Model file for the job. Use its own axes, mm. Face numbers are marked on the shaded views. Round coordinates to 2 decimals unless told otherwise and drop trailing zeros. Order: outer loops, then holes, each group sorted by start corner. A loop starts at its lowest first (then second) coordinate and runs counter-clockwise, first axis right, second up. Notation, with made-up numbers: (-10.75, 84) -> (21.25, 84) arc R21 ccw to (21.25, 112) -> close; hole circle Ø11 at (64.25, 3). An arc over 180 degrees is marked (long way). Put each result on its own line as item: value. Start each with the question number.
Q1. Pull direction Y, two halves, no side cores. Call the marked faces 1, 2, 3 and 4: released by +Y, released by -Y, zero draft, split by the parting line, or undercut.
Q2. Cut at D-D, the plane z = 47.5. List the corners of the cut face in (x, y), and give its area (3 significant figures).
Q3. Cut at B-B, the plane x = 7.5. List the corners of the cut face in (y, z), and give its area (3 significant figures).
Q4. Cut at A-A, the plane z = 43.25. List the corners of the cut face in (x, y), and give its area (3 significant figures).
Q5. Cut at C-C, the plane y = 3.45. List the corners of the cut face in (x, z).
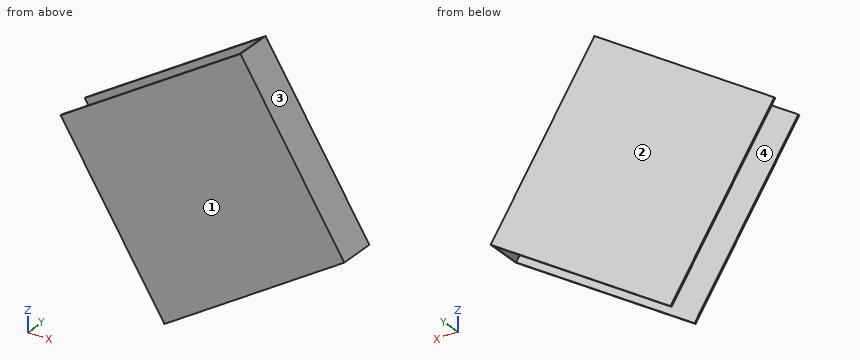
from build123d import *

# Parameters (mm, degrees)
BOX163_W               = 6
BOX163_H               = 6.45
BOX163_DEPTH           = 1.05
BOX162_W               = 6
BOX162_H               = 6.5
BOX162_DEPTH           = 1.15
CUT079_ROLL_ANGLE      = 90
CUT079_PITCH_ANGLE     = -58
CUT079_PLACEMENT_ANGLE = 180


with BuildPart() as small_cu_gnd_electrode068:
    # Box163 → Box163 (new body)
    with BuildSketch(Plane.XY.offset(0.05)):
        with Locations((3, 3.225)):
            Rectangle(BOX163_W, BOX163_H)
    extrude(amount=BOX163_DEPTH)


with BuildPart() as small_cu_electrode002_short_axis_gnd007:
    # Box162 → Box162 (new body)
    with BuildSketch(Plane.XY):
        with Locations((3, 3.25)):
            Rectangle(BOX162_W, BOX162_H)
    extrude(amount=BOX162_DEPTH)

    # Cut079: cut Small Cu GND Electrode068
    add(small_cu_gnd_electrode068.part, mode=Mode.SUBTRACT)


with BuildPart() as small_cu_electrode002_short_axis_gnd007_1:
    # Cut079 roll: moved
    add(small_cu_electrode002_short_axis_gnd007.part.rotate(Axis((0, 0, 0), (1, 0, 0)), CUT079_ROLL_ANGLE))


with BuildPart() as small_cu_electrode002_short_axis_gnd007_2:
    # Cut079 pitch: moved
    add(small_cu_electrode002_short_axis_gnd007_1.part.rotate(Axis((0, 0, 0), (0, 1, 0)), CUT079_PITCH_ANGLE))


with BuildPart() as small_cu_electrode002_short_axis_gnd007_3:
    # Cut079 placement: moved
    add(small_cu_electrode002_short_axis_gnd007_2.part.moved(Location((9.199953, 2.74, 40.788858))).rotate(Axis((9.199953, 2.74, 40.788858), (0, 0, 1)), CUT079_PLACEMENT_ANGLE))


solid = small_cu_electrode002_short_axis_gnd007_3.part
Ans:
1. face 1: released by -Y
1. face 2: released by +Y
1. face 3: zero draft
1. face 4: undercut
2. outline: (8.62, 2.74) -> (12.67, 2.74) -> (12.67, 3.89) -> (8.62, 3.89) -> (8.62, 3.84) -> (12.61, 3.84) -> (12.61, 2.79) -> (8.62, 2.79) -> close
2. area: 0.467 mm^2
3. outline: (2.74, 43.51) -> (2.79, 43.51) -> (2.79, 46.8) -> (2.74, 46.8) -> close; (3.84, 43.51) -> (3.89, 43.51) -> (3.89, 46.8) -> (3.84, 46.8) -> close
3. area: 0.329 mm^2
4. outline: (7.66, 2.74) -> (13.14, 2.74) -> (13.14, 2.79) -> (7.66, 2.79) -> close; (7.66, 3.84) -> (13.14, 3.84) -> (13.14, 3.89) -> (7.66, 3.89) -> close
4. area: 0.548 mm^2
5. outline: (11.49, 49.3) -> (14.67, 44.21) -> (14.71, 44.23) -> (11.53, 49.32) -> close
